Geometry: final body of the model. Coordinates: model frame, mm. Give positions to 0.01 mm unless a question says otherwise; leave off trailing zeros. Order: outer loops, then holes, each group sorted by start corner. A loop starts at its lowest first (then second) coordinate and runs counter-clockwise, first axis right, second up. Notation, with made-up numbers: (11.5, 71.25) - (67.5, 71.25) arc R33 cw to (67.5, 99.25) - close; hole circle Ø10 at (51, 79). An arc over 180 degrees is marked (long way). One line per item, written item: value.
```python
from build123d import *

# Parameters (mm, degrees)
SKETCH1_W           = 4.1
SKETCH1_H           = 1.7
SKETCH1_W_2         = 1.7
SKETCH1_H_2         = 4.1
BOSS_EXTRUDE1_DEPTH = 2
CUT_EXTRUDE1_REACH  = 51.538
SKETCH2_R           = 1.6
CUT_EXTRUDE2_REACH  = 51.538
SKETCH4_R           = 0.5
CUT_EXTRUDE3_DEPTH  = 2
CUT_EXTRUDE4_REACH  = 51.538
SKETCH5_R           = 1.6


with BuildPart() as part:
    # Sketch1 → Boss-Extrude1 (new body)
    with BuildSketch(Plane.XY):
        Polygon((-14.497474683, 35), (14.497474683, 35), (35, 14.497474683), (35, -14.497474683), (14.497474683, -35), (-14.497474683, -35), (-35, -14.497474683), (-35, 14.497474683), align=None)
        with Locations((-23, 5.8)):
            Rectangle(SKETCH1_W, SKETCH1_H, mode=Mode.SUBTRACT)
        with Locations((5.8, 23)):
            Rectangle(SKETCH1_W_2, SKETCH1_H_2, mode=Mode.SUBTRACT)
        with Locations((-23, -5.8)):
            Rectangle(SKETCH1_W, SKETCH1_H, mode=Mode.SUBTRACT)
        with Locations((-5.8, 23)):
            Rectangle(SKETCH1_W_2, SKETCH1_H_2, mode=Mode.SUBTRACT)
        with Locations((23, -5.8)):
            Rectangle(SKETCH1_W, SKETCH1_H, mode=Mode.SUBTRACT)
        with Locations((23, 5.8)):
            Rectangle(SKETCH1_W, SKETCH1_H, mode=Mode.SUBTRACT)
        with Locations((-5.8, -23)):
            Rectangle(SKETCH1_W_2, SKETCH1_H_2, mode=Mode.SUBTRACT)
        with Locations((5.8, -23)):
            Rectangle(SKETCH1_W_2, SKETCH1_H_2, mode=Mode.SUBTRACT)
    extrude(amount=BOSS_EXTRUDE1_DEPTH)

    # Sketch2 → Cut-Extrude1 (cut, up to next)
    with BuildSketch(Plane.XY.offset(2), mode=Mode.PRIVATE) as cut_extrude1_sk1:
        with Locations((-23, 0)):
            Circle(SKETCH2_R)
    cut_extrude1_tool1 = extrude(cut_extrude1_sk1.sketch, amount=-CUT_EXTRUDE1_REACH, mode=Mode.PRIVATE) & part.part
    # Sketch2 → Cut-Extrude1 (cut, up to next)
    with BuildSketch(Plane.XY.offset(2), mode=Mode.PRIVATE) as cut_extrude1_sk2:
        with Locations((0, 23)):
            Circle(SKETCH2_R)
    cut_extrude1_tool2 = extrude(cut_extrude1_sk2.sketch, amount=-CUT_EXTRUDE1_REACH, mode=Mode.PRIVATE) & part.part
    # Sketch2 → Cut-Extrude1 (cut, up to next)
    with BuildSketch(Plane.XY.offset(2), mode=Mode.PRIVATE) as cut_extrude1_sk3:
        with Locations((23, 0)):
            Circle(SKETCH2_R)
    cut_extrude1_tool3 = extrude(cut_extrude1_sk3.sketch, amount=-CUT_EXTRUDE1_REACH, mode=Mode.PRIVATE) & part.part
    # Sketch2 → Cut-Extrude1 (cut, up to next)
    with BuildSketch(Plane.XY.offset(2), mode=Mode.PRIVATE) as cut_extrude1_sk4:
        with Locations((0, -23)):
            Circle(SKETCH2_R)
    cut_extrude1_tool4 = extrude(cut_extrude1_sk4.sketch, amount=-CUT_EXTRUDE1_REACH, mode=Mode.PRIVATE) & part.part
    add(cut_extrude1_tool1.solids().sort_by_distance((-23, 0, 2))[0], mode=Mode.SUBTRACT)
    add(cut_extrude1_tool2.solids().sort_by_distance((0, 23, 2))[0], mode=Mode.SUBTRACT)
    add(cut_extrude1_tool3.solids().sort_by_distance((23, 0, 2))[0], mode=Mode.SUBTRACT)
    add(cut_extrude1_tool4.solids().sort_by_distance((0, -23, 2))[0], mode=Mode.SUBTRACT)

    # Sketch3 → Cut-Extrude2 (cut, up to next)
    with BuildSketch(Plane.XY.offset(2), mode=Mode.PRIVATE) as cut_extrude2_sk1:
        with BuildLine():
            Line((-32.244069222, -1.697056275), (-28.708535316, 1.838477631))
            ThreePointArc((-28.708535316, 1.838477631), (-28.708535316, 2.545584412), (-28.001428535, 2.545584412))
            Line((-28.001428535, 2.545584412), (-26.870057685, 1.414213562))
            ThreePointArc((-26.870057685, 1.414213562), (-26.870057685, 0.707106781), (-27.577164466, 0.707106781))
            Line((-27.577164466, 0.707106781), (-31.112698372, -2.828427125))
            ThreePointArc((-31.112698372, -2.828427125), (-31.112698372, -3.535533906), (-31.819805153, -3.535533906))
            Line((-31.819805153, -3.535533906), (-32.951176003, -2.404163056))
            ThreePointArc((-32.951176003, -2.404163056), (-32.951176003, -1.697056275), (-32.244069222, -1.697056275))
        make_face()
    cut_extrude2_tool1 = extrude(cut_extrude2_sk1.sketch, amount=-CUT_EXTRUDE2_REACH, mode=Mode.PRIVATE) & part.part
    # Sketch3 → Cut-Extrude2 (cut, up to next)
    with BuildSketch(Plane.XY.offset(2), mode=Mode.PRIVATE) as cut_extrude2_sk2:
        with BuildLine():
            Line((-3.535533906, -31.819805153), (-2.404163056, -32.951176003))
            ThreePointArc((-2.404163056, -32.951176003), (-1.697056275, -32.951176003), (-1.697056275, -32.244069222))
            Line((-1.697056275, -32.244069222), (1.838477631, -28.708535316))
            ThreePointArc((1.838477631, -28.708535316), (2.545584412, -28.708535316), (2.545584412, -28.001428535))
            Line((2.545584412, -28.001428535), (1.414213562, -26.870057685))
            ThreePointArc((1.414213562, -26.870057685), (0.707106781, -26.870057685), (0.707106781, -27.577164466))
            Line((0.707106781, -27.577164466), (-2.828427125, -31.112698372))
            ThreePointArc((-2.828427125, -31.112698372), (-3.535533906, -31.112698372), (-3.535533906, -31.819805153))
        make_face()
    cut_extrude2_tool2 = extrude(cut_extrude2_sk2.sketch, amount=-CUT_EXTRUDE2_REACH, mode=Mode.PRIVATE) & part.part
    # Sketch3 → Cut-Extrude2 (cut, up to next)
    with BuildSketch(Plane.XY.offset(2), mode=Mode.PRIVATE) as cut_extrude2_sk3:
        with BuildLine():
            Line((32.244069222, 1.697056275), (28.708535316, -1.838477631))
            ThreePointArc((28.708535316, -1.838477631), (28.708535316, -2.545584412), (28.001428535, -2.545584412))
            Line((28.001428535, -2.545584412), (26.870057685, -1.414213562))
            ThreePointArc((26.870057685, -1.414213562), (26.870057685, -0.707106781), (27.577164466, -0.707106781))
            Line((27.577164466, -0.707106781), (31.112698372, 2.828427125))
            ThreePointArc((31.112698372, 2.828427125), (31.112698372, 3.535533906), (31.819805153, 3.535533906))
            Line((31.819805153, 3.535533906), (32.951176003, 2.404163056))
            ThreePointArc((32.951176003, 2.404163056), (32.951176003, 1.697056275), (32.244069222, 1.697056275))
        make_face()
    cut_extrude2_tool3 = extrude(cut_extrude2_sk3.sketch, amount=-CUT_EXTRUDE2_REACH, mode=Mode.PRIVATE) & part.part
    # Sketch3 → Cut-Extrude2 (cut, up to next)
    with BuildSketch(Plane.XY.offset(2), mode=Mode.PRIVATE) as cut_extrude2_sk4:
        with BuildLine():
            Line((3.535533906, 31.819805153), (2.404163056, 32.951176003))
            ThreePointArc((2.404163056, 32.951176003), (1.697056275, 32.951176003), (1.697056275, 32.244069222))
            Line((1.697056275, 32.244069222), (-1.838477631, 28.708535316))
            ThreePointArc((-1.838477631, 28.708535316), (-2.545584412, 28.708535316), (-2.545584412, 28.001428535))
            Line((-2.545584412, 28.001428535), (-1.414213562, 26.870057685))
            ThreePointArc((-1.414213562, 26.870057685), (-0.707106781, 26.870057685), (-0.707106781, 27.577164466))
            Line((-0.707106781, 27.577164466), (2.828427125, 31.112698372))
            ThreePointArc((2.828427125, 31.112698372), (3.535533906, 31.112698372), (3.535533906, 31.819805153))
        make_face()
    cut_extrude2_tool4 = extrude(cut_extrude2_sk4.sketch, amount=-CUT_EXTRUDE2_REACH, mode=Mode.PRIVATE) & part.part
    add(cut_extrude2_tool1.solids().sort_by_distance((-29.910617, -0.494975, 2))[0], mode=Mode.SUBTRACT)
    add(cut_extrude2_tool2.solids().sort_by_distance((-0.494975, -29.910617, 2))[0], mode=Mode.SUBTRACT)
    add(cut_extrude2_tool3.solids().sort_by_distance((29.910617, 0.494975, 2))[0], mode=Mode.SUBTRACT)
    add(cut_extrude2_tool4.solids().sort_by_distance((0.494975, 29.910617, 2))[0], mode=Mode.SUBTRACT)

    # Sketch4 → Cut-Extrude3 (cut)
    with BuildSketch(Plane.XY.offset(2)):
        with Locations((-24.55, 6.65)):
            Circle(SKETCH4_R)
        with Locations((-24.55, 4.95)):
            Circle(SKETCH4_R)
        with Locations((-21.45, 6.65)):
            Circle(SKETCH4_R)
        with Locations((-21.45, 4.95)):
            Circle(SKETCH4_R)
        with Locations((-21.45, -4.95)):
            Circle(SKETCH4_R)
        with Locations((-21.45, -6.65)):
            Circle(SKETCH4_R)
        with Locations((-24.55, -4.95)):
            Circle(SKETCH4_R)
        with Locations((-24.55, -6.65)):
            Circle(SKETCH4_R)
        with Locations((6.65, 24.55)):
            Circle(SKETCH4_R)
        with Locations((4.95, 24.55)):
            Circle(SKETCH4_R)
        with Locations((6.65, 21.45)):
            Circle(SKETCH4_R)
        with Locations((4.95, 21.45)):
            Circle(SKETCH4_R)
        with Locations((-4.95, 21.45)):
            Circle(SKETCH4_R)
        with Locations((-6.65, 21.45)):
            Circle(SKETCH4_R)
        with Locations((-4.95, 24.55)):
            Circle(SKETCH4_R)
        with Locations((-6.65, 24.55)):
            Circle(SKETCH4_R)
        with Locations((24.55, -6.65)):
            Circle(SKETCH4_R)
        with Locations((24.55, -4.95)):
            Circle(SKETCH4_R)
        with Locations((21.45, -6.65)):
            Circle(SKETCH4_R)
        with Locations((21.45, -4.95)):
            Circle(SKETCH4_R)
        with Locations((21.45, 4.95)):
            Circle(SKETCH4_R)
        with Locations((21.45, 6.65)):
            Circle(SKETCH4_R)
        with Locations((24.55, 4.95)):
            Circle(SKETCH4_R)
        with Locations((24.55, 6.65)):
            Circle(SKETCH4_R)
        with Locations((-6.65, -24.55)):
            Circle(SKETCH4_R)
        with Locations((-4.95, -24.55)):
            Circle(SKETCH4_R)
        with Locations((-6.65, -21.45)):
            Circle(SKETCH4_R)
        with Locations((-4.95, -21.45)):
            Circle(SKETCH4_R)
        with Locations((4.95, -21.45)):
            Circle(SKETCH4_R)
        with Locations((6.65, -21.45)):
            Circle(SKETCH4_R)
        with Locations((4.95, -24.55)):
            Circle(SKETCH4_R)
        with Locations((6.65, -24.55)):
            Circle(SKETCH4_R)
    extrude(amount=-CUT_EXTRUDE3_DEPTH, mode=Mode.SUBTRACT)

    # Sketch5 → Cut-Extrude4 (cut, up to next)
    with BuildSketch(Plane.XY.offset(2), mode=Mode.PRIVATE) as cut_extrude4_sk1:
        with Locations((-14.707821049, 14.707821049)):
            Circle(SKETCH5_R)
    cut_extrude4_tool1 = extrude(cut_extrude4_sk1.sketch, amount=-CUT_EXTRUDE4_REACH, mode=Mode.PRIVATE) & part.part
    # Sketch5 → Cut-Extrude4 (cut, up to next)
    with BuildSketch(Plane.XY.offset(2), mode=Mode.PRIVATE) as cut_extrude4_sk2:
        with Locations((14.707821049, -14.707821049)):
            Circle(SKETCH5_R)
    cut_extrude4_tool2 = extrude(cut_extrude4_sk2.sketch, amount=-CUT_EXTRUDE4_REACH, mode=Mode.PRIVATE) & part.part
    add(cut_extrude4_tool1.solids().sort_by_distance((-14.707821, 14.707821, 2))[0], mode=Mode.SUBTRACT)
    add(cut_extrude4_tool2.solids().sort_by_distance((14.707821, -14.707821, 2))[0], mode=Mode.SUBTRACT)


solid = part.part
```
1) First-contact query: pin 1 (1 mm diameter, centred on y = -22.5, z = 0.5, fed in from -X); pin 2 (0.6 mm diameter, centred on y = -22.5, z = 1.5, fed in from +X); pin 3 (1 mm diameter, centred on x = 22.5, z = 0.5, fed in from -Y). Flat tips, straight axial feed; report the tip coordinate or a pass-through.
Answers below:
pin 1: x = -27.5
pin 2: x = 27.3
pin 3: y = -27.5
2) Section B-B, the plane x = 18. Return loops of the section in (y, z), then the cut area to 3 significant figures.
Answers below:
outline: (-31.5, 0) - (31.5, 0) - (31.5, 2) - (-31.5, 2) - close
area: 126 mm^2
3) Material intervals for line 1 along Y through (x, z) = (0, 1.1); line 2 along Y through (x, z) = (-23, 1); line 3 along Y through (x, z) = (-14, 0.35), sorted ascending.
Answers below:
line 1: -35 to -30.55, -28.28 to -24.6, -21.4 to 21.4, 24.6 to 28.28, 30.55 to 35
line 2: -26.5 to -6.65, -4.95 to -1.6, 1.6 to 4.95, 6.65 to 26.5
line 3: -35 to 13.27, 16.14 to 35
4) Mould query, pull axis X, two halves, no side actions, for faces 1 (the face through (4.95, 23, 1)), 2 (the face through (-35, 0, 1)), 3 (the face through (24.9, -24.6, 1)). Classes: released by +X, released by -X, zero draft, split by the parting line, or undercut.
Answers below:
face 1: undercut
face 2: released by -X
face 3: released by +X
5) Section A-A, the plane z = 0.7. Count the separate pieces of the cut face and the enclosed holes in it, then the cut area to 3 significant figures.
Answers below:
separate pieces: 1
enclosed holes: 18
area: 3,890 mm^2
